from build123d import *

# Parameters (mm, degrees)
SALIENTE_EXTRUIR1_DEPTH          = 10
TALADRO_DE_MARGEN_PARA_M41_D     = 4.5
TALADRO_DE_MARGEN_PARA_M41_DEPTH = 10
TALADRO_DE_MARGEN_PARA_M41_TIP   = 1.351936393
TALADRO_DE_MARGEN_PARA_M42_D     = 4.5
TALADRO_DE_MARGEN_PARA_M42_DEPTH = 10
TALADRO_DE_MARGEN_PARA_M42_TIP   = 1.351936393


with BuildPart() as part:
    # Croquis1 → Saliente-Extruir1 (new body)
    with BuildSketch(Plane.XY):
        Polygon((40, -8), (8, -40), (0, -40), (0, 0), (40, 0), align=None)
    extrude(amount=SALIENTE_EXTRUIR1_DEPTH)

    # Taladro de margen para M41
    with Locations(Plane(origin=(0, 0, 0), x_dir=(1, 0, 0), z_dir=(0, 1, 0))):
        with Locations((12, -5), (32, -5)):
            Hole(TALADRO_DE_MARGEN_PARA_M41_D / 2, depth=TALADRO_DE_MARGEN_PARA_M41_DEPTH)
            with Locations((0, 0, -(TALADRO_DE_MARGEN_PARA_M41_DEPTH + TALADRO_DE_MARGEN_PARA_M41_TIP / 2))):  # 118° drill point
                Cone(0, TALADRO_DE_MARGEN_PARA_M41_D / 2, TALADRO_DE_MARGEN_PARA_M41_TIP, mode=Mode.SUBTRACT)

    # Taladro de margen para M42
    with Locations(Plane.ZY):
        with Locations((5, -12), (5, -32)):
            Hole(TALADRO_DE_MARGEN_PARA_M42_D / 2, depth=TALADRO_DE_MARGEN_PARA_M42_DEPTH)
            with Locations((0, 0, -(TALADRO_DE_MARGEN_PARA_M42_DEPTH + TALADRO_DE_MARGEN_PARA_M42_TIP / 2))):  # 118° drill point
                Cone(0, TALADRO_DE_MARGEN_PARA_M42_D / 2, TALADRO_DE_MARGEN_PARA_M42_TIP, mode=Mode.SUBTRACT)


solid = part.part
Here's how the part is built. I have some questions about the finished solid (model axes, mm). A direction names the side the tool comes from. Coordinates: 2 decimals unless noted, no trailing zeros. Write each loop counter-clockwise with the first axis right and the second up, starting at its lowest first coordinate (ties: lowest second). Pieces come first, ordered by that corner, then holes.
Item 1: On a 3-axis mill with a long thin cutter (end or side, diameter ignored), from which of +Z, -Z, +X, -X, +Y, -Y can I reach the whole of each face in a straight line? I mean faces 5 (the cylindrical face through (14.248, -5.07, 4.901)), 6 (the cylindrical face through (5.07, -10.103, 3.79)), 7 (the flat face through (4, -40, 5)). Say none if no direction works.
Item 2: I want a section at A-A on x = 6. Write out the boundary of the cut face in (y, z), and give its area (3 significant figures).
Item 3: Will these pins go through, and if not, where does the flat tip stop? pin 1 (5 mm diameter, centred on x = 32, z = 5, fed in from -Y); pin 2 (4 mm diameter, centred on y = -32, z = 5, fed in from +X); pin 3 (4 mm diameter, centred on x = 12, z = 5, fed in from -Y); pin 4 (2 mm diameter, centred on x = 18.5, y = -31, fed in from -Z).
Item 4: I want a section at D-D on y = -27. Write out the boundary of the cut face in (x, z), and give its area (3 significant figures).
Item 5: I want a section at C-C on z = 9.25. Write out the boundary of the cut face in (x, y), and give its area (3 significant figures).
Item 6: If we mould it in two halves opening along Z, with no side actions, what happens to faces 1 (the flat face through (16, -15, 0)), 2 (the conical face through (11.12, -12.38, 4.92)), 3 (the flat face through (20, 0, 5)), 4 (the conical face through (31.71, -11.12, 4.74))? For each: +Z half, -Z half, draft (parallel to the pull), parting line (faces both ways), or undercut.
Item 7: I want a section at B-B on y = -4. Write out the boundary of the cut face in (x, z).
Item 8: If I drill on line 1 (Y direction, x = 2.75, z = 5); line 2 (Z direction, x = 4, y = -12); line 3 (X direction, y = -6.5, z = 4), over which ranges is the centre line in solid material (lowest first)?
Findings below:
1. face 5: +Y
1. face 6: -X
1. face 7: +Z, -Z, +X, -X, -Y
2. outline: (-40, 0) - (0, 0) - (0, 10) - (-40, 10) - close; hole circle Ø4.5 at (-32, 5); hole circle Ø4.5 at (-12, 5)
2. area: 368 mm2
3. pin 1: stops at y = -18.5
3. pin 2: stops at x = 18
3. pin 3: stops at y = -38
3. pin 4: passes through
4. outline: (0, 0) - (21, 0) - (21, 10) - (0, 10) - close
4. area: 210 mm2
5. outline: (0, -40) - (8, -40) - (40, -8) - (40, 0) - (0, 0) - close
5. area: 1,090 mm2
6. face 1: -Z half
6. face 2: undercut
6. face 3: draft
6. face 4: undercut
7. outline: (0, 0) - (40, 0) - (40, 10) - (0, 10) - close; hole circle Ø4.5 at (12, 5); hole circle Ø4.5 at (32, 5)
8. line 1: y = -40 to -34.25, -29.75 to -14.25, -9.75 to 0
8. line 2: z = 0 to 2.75, 7.25 to 10
8. line 3: x = 0 to 9.98, 14.02 to 29.98, 34.02 to 40
